CAD build for the part. Positions are in the model's coordinates, mm. Give positions to 0.01 mm unless a question says otherwise; leave off trailing zeros. Loops run counter-clockwise (first coordinate to the right, second up) from the corner with the lowest first, then second, coordinate; pieces in that order, holes last. Notation, with made-up numbers: M -39,-13 L -16,-13 A12 ccw -16,4 Z; hole C -23.5,45.25 d10. An arc over 180 degrees is marked long. Answer as CSV lines item,"result".
from build123d import *

# Parameters (mm, degrees)
SKETCH2_R                = 95.25
BOSS_EXTRUDE1_DEPTH      = 387.35
SKETCH6_R                = 95.25
F_7_PERCENT_ULLAGE_DEPTH = 57.15


with BuildPart() as part:
    # Sketch2 → Boss-Extrude1 (new body)
    with BuildSketch(Plane(origin=(0, 0, 0), x_dir=(1, 0, 0), z_dir=(0, 1, 0))):
        Circle(SKETCH2_R)
    extrude(amount=BOSS_EXTRUDE1_DEPTH)

    # Sketch3 → Revolve2 (revolve)
    with BuildSketch(Plane(origin=(0, 0, 0), x_dir=(0, 0, -1), z_dir=(1, 0, 0))):
        with BuildLine():
            Line((0, 447.04), (0, 387.35))
            Line((0, 387.35), (95.25, 387.35))
            add(Edge.make_bspline(
                [(95.25, 387.35), (95.25, 447.04), (0, 447.04)],
                knots=[3.141592654, 3.141592654, 3.141592654, 4.71238898, 4.71238898, 4.71238898], degree=2, weights=[1, 0.707106781, 1]))
        make_face()
    revolve(axis=Axis((0, 447.04, 0), (0, -1, 0)))

    # Sketch4 → Revolve3 (revolve)
    with BuildSketch(Plane(origin=(0, 0, 0), x_dir=(0, 0, -1), z_dir=(1, 0, 0))):
        with BuildLine():
            Line((0, -61.214), (0, 0))
            Line((0, 0), (95.25, 0))
            add(Edge.make_bspline(
                [(0, -61.214), (95.25, -61.214), (95.25, 0)],
                knots=[4.71238898, 4.71238898, 4.71238898, 6.283185307, 6.283185307, 6.283185307], degree=2, weights=[1, 0.707106781, 1]))
        make_face()
    revolve(axis=Axis((0, -61.214, 0), (0, 1, 0)))

    # Sketch6 → 7 Percent Ullage (cut)
    with BuildSketch(Plane(origin=(0, 447.04, 0), x_dir=(1, 0, 0), z_dir=(0, 1, 0))):
        Circle(SKETCH6_R)
    extrude(amount=-F_7_PERCENT_ULLAGE_DEPTH, mode=Mode.SUBTRACT)


solid = part.part
1) Flat gauge pins, fed straight in: pin 1 (8 mm diameter, centred on x = -9.5, y = 95, fed in from -Z); pin 2 (2 mm diameter, centred on x = 47.5, z = 4, fed in from -Y); pin 3 (8 mm diameter, centred on x = 72.5, y = 258.5, fed in from -Z). Where does each tip first touch, or does it go through?
Answer below:
pin 1,"stops at z = -95.09"
pin 2,"stops at y = -53.36"
pin 3,"stops at z = -66.18"
2) Drill centre lines: line 1 (Z direction, x = 1.5, y = 205); line 2 (Z direction, x = 5.5, y = 94.5); line 3 (Y direction, x = -80, z = -16). Where is each one in solid material? Low to high. Write a range as from..to.
Answer below:
line 1,"z = -95.24..95.24"
line 2,"z = -95.09..95.09"
line 3,"y = -31.59..389.89"
3) Band-saw the part on A-A on y = 11. Give the cut face in (x, z), and give its area (3 significant figures).
Answer below:
outline,"C 0,0 d190.5"
area,"28,500 mm^2"
